```python
from build123d import *

# Parameters (mm, degrees)
SKETCH1_W          = 520
SKETCH1_H          = 192.12
BASE_FLANGE1_DEPTH = 3.26
SKETCH2_R          = 4.5
CUT_EXTRUDE1_DEPTH = 10
SKETCH3_R          = 2.5
CUT_EXTRUDE2_DEPTH = 10
SKETCH4_R          = 2.5
CUT_EXTRUDE3_DEPTH = 10
FILLET2_R          = 5
CHAMFER1_SIZE      = 2.5


# Sheet-metal steps are written as plain solids
with BuildPart() as part:
    # Sketch1 → Base-Flange1 (new body)
    with BuildSketch(Plane(origin=(0, 0, 0), x_dir=(1, 0, 0), z_dir=(0, 1, 0))):
        with Locations((0, -0.985)):
            Rectangle(SKETCH1_W, SKETCH1_H)
    extrude(amount=-BASE_FLANGE1_DEPTH)

    # Sketch2 → Cut-Extrude1 (cut)
    with BuildSketch(Plane(origin=(0, 0, 0), x_dir=(1, 0, 0), z_dir=(0, 1, 0))):
        with Locations(Location((130, 80.075, 0), (0, 0, 270))):
            Circle(SKETCH2_R)
        with Locations(Location((130, -82.545, 0), (0, 0, 270))):
            Circle(SKETCH2_R)
        with Locations(Location((-130, 80.075, 0), (0, 0, 270))):
            Circle(SKETCH2_R)
        with Locations(Location((-130, -82.545, 0), (0, 0, 270))):
            Circle(SKETCH2_R)
    extrude(amount=-CUT_EXTRUDE1_DEPTH, mode=Mode.SUBTRACT)

    # Sketch3 → Cut-Extrude2 (cut)
    with BuildSketch(Plane(origin=(0, 0, 0), x_dir=(1, 0, 0), z_dir=(0, 1, 0))):
        with Locations(Location((-52.5, 52.5, 0), (0, 0, 270))):
            Circle(SKETCH3_R)
        with Locations(Location((52.5, 52.5, 0), (0, 0, 270))):
            Circle(SKETCH3_R)
        with Locations(Location((52.5, -52.5, 0), (0, 0, 270))):
            Circle(SKETCH3_R)
        with Locations(Location((-52.5, -52.5, 0), (0, 0, 270))):
            Circle(SKETCH3_R)
        with BuildLine():
            Line((-3, -59.924953066), (-3, -19.773719933))
            ThreePointArc((-3, -19.773719933), (-7.653668647, -18.47759065), (-11.860811111, -16.103451798))
            Line((-11.860811111, -16.103451798), (-40.252020332, -44.494661019))
            ThreePointArc((-40.252020332, -44.494661019), (-22.961005942, -55.432771951), (-3, -59.924953066))
        make_face()
        with BuildLine():
            Line((-3, 59.924953066), (-3, 19.773719933))
            ThreePointArc((-3, 19.773719933), (-7.653668647, 18.47759065), (-11.860811111, 16.103451798))
            Line((-11.860811111, 16.103451798), (-40.252020332, 44.494661019))
            ThreePointArc((-40.252020332, 44.494661019), (-22.961005942, 55.432771951), (-3, 59.924953066))
        make_face()
        with BuildLine():
            Line((-19.773719933, 3), (-59.924953066, 3))
            ThreePointArc((-59.924953066, 3), (-55.432771951, 22.961005942), (-44.494661019, 40.252020332))
            Line((-44.494661019, 40.252020332), (-16.103451798, 11.860811111))
            ThreePointArc((-16.103451798, 11.860811111), (-18.47759065, 7.653668647), (-19.773719933, 3))
        make_face()
        with BuildLine():
            Line((-19.773719933, -3), (-59.924953066, -3))
            ThreePointArc((-59.924953066, -3), (-55.432771951, -22.961005942), (-44.494661019, -40.252020332))
            Line((-44.494661019, -40.252020332), (-16.103451798, -11.860811111))
            ThreePointArc((-16.103451798, -11.860811111), (-18.47759065, -7.653668647), (-19.773719933, -3))
        make_face()
        with BuildLine():
            Line((3, -59.924953066), (3, -19.773719933))
            ThreePointArc((3, -19.773719933), (7.653668647, -18.47759065), (11.860811111, -16.103451798))
            Line((11.860811111, -16.103451798), (40.252020332, -44.494661019))
            ThreePointArc((40.252020332, -44.494661019), (22.961005942, -55.432771951), (3, -59.924953066))
        make_face()
        with BuildLine():
            Line((44.494661019, -40.252020332), (16.103451798, -11.860811111))
            ThreePointArc((16.103451798, -11.860811111), (18.47759065, -7.653668647), (19.773719933, -3))
            Line((19.773719933, -3), (59.924953066, -3))
            ThreePointArc((59.924953066, -3), (55.432771951, -22.961005942), (44.494661019, -40.252020332))
        make_face()
        with BuildLine():
            Line((19.773719933, 3), (59.924953066, 3))
            ThreePointArc((59.924953066, 3), (55.432771951, 22.961005942), (44.494661019, 40.252020332))
            Line((44.494661019, 40.252020332), (16.103451798, 11.860811111))
            ThreePointArc((16.103451798, 11.860811111), (18.47759065, 7.653668647), (19.773719933, 3))
        make_face()
        with BuildLine():
            Line((40.252020332, 44.494661019), (11.860811111, 16.103451798))
            ThreePointArc((11.860811111, 16.103451798), (7.653668647, 18.47759065), (3, 19.773719933))
            Line((3, 19.773719933), (3, 59.924953066))
            ThreePointArc((3, 59.924953066), (22.961005942, 55.432771951), (40.252020332, 44.494661019))
        make_face()
    extrude(amount=-CUT_EXTRUDE2_DEPTH, mode=Mode.SUBTRACT)

    # Sketch4 → Cut-Extrude3 (cut)
    with BuildSketch(Plane(origin=(0, 0, 0), x_dir=(1, 0, 0), z_dir=(0, 1, 0))):
        with Locations(Location((-92.5, 52.5, 0), (0, 0, 270))):
            Circle(SKETCH4_R)
        with Locations(Location((-197.5, 52.5, 0), (0, 0, 270))):
            Circle(SKETCH4_R)
        with Locations(Location((-197.5, -52.5, 0), (0, 0, 270))):
            Circle(SKETCH4_R)
        with Locations(Location((-92.5, -52.5, 0), (0, 0, 270))):
            Circle(SKETCH4_R)
        with Locations(Location((92.5, -52.5, 0), (0, 0, 270))):
            Circle(SKETCH4_R)
        with Locations(Location((197.5, -52.5, 0), (0, 0, 270))):
            Circle(SKETCH4_R)
        with Locations(Location((197.5, 52.5, 0), (0, 0, 270))):
            Circle(SKETCH4_R)
        with Locations(Location((92.5, 52.5, 0), (0, 0, 270))):
            Circle(SKETCH4_R)
        Polygon((-100, 60), (-190, 60), (-190, 45), (-205, 45), (-205, -45), (-190, -45), (-190, -60), (-100, -60), (-100, -45), (-85, -45), (-85, 45), (-100, 45), align=None)
        Polygon((100, 45), (100, 60), (190, 60), (190, 45), (205, 45), (205, -45), (190, -45), (190, -60), (100, -60), (100, -45), (85, -45), (85, 45), align=None)
    extrude(amount=-CUT_EXTRUDE3_DEPTH, mode=Mode.SUBTRACT)

    # Fillet2
    fillet2_edges = [part.edges().sort_by_distance(p)[0] for p in [
        (-100, -1.63, -60),
        (-100, -1.63, -45),
        (-85, -1.63, -45),
        (-85, -1.63, 45),
        (-100, -1.63, 45),
        (-100, -1.63, 60),
        (-190, -1.63, 60),
        (-190, -1.63, 45),
        (-205, -1.63, 45),
        (-205, -1.63, -45),
        (-190, -1.63, -45),
        (-190, -1.63, -60),
        (85, -1.63, -45),
        (100, -1.63, -45),
        (100, -1.63, -60),
        (190, -1.63, -60),
        (190, -1.63, -45),
        (205, -1.63, -45),
        (205, -1.63, 45),
        (190, -1.63, 45),
        (190, -1.63, 60),
        (100, -1.63, 60),
        (100, -1.63, 45),
        (85, -1.63, 45),
    ]]
    fillet(fillet2_edges, radius=FILLET2_R)

    # Chamfer1
    chamfer1_edges = [part.edges().sort_by_distance(p)[0] for p in [
        (130, 0, -84.575),
        (130, 0, 78.045),
        (-130, 0, -84.575),
        (-130, 0, 78.045),
    ]]
    chamfer(chamfer1_edges, length=CHAMFER1_SIZE)


solid = part.part
```
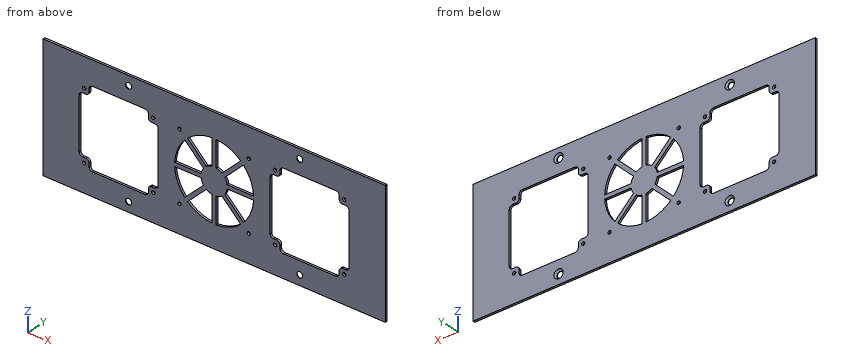
Here's how the part is built. I have some questions about the finished solid (model axes, mm). Coordinates: 2 decimals unless noted, no trailing zeros. Order: outer loops, then holes, each group sorted by start corner. A loop starts at its lowest first (then second) coordinate and runs counter-clockwise, first axis right, second up. Notation, with made-up numbers: (73, 25) -> (96, 25) arc R14 cw to (96, 34) -> close; hole circle Ø1 at (18.25, 21). An arc over 180 degrees is marked (long way). Return JSON: item names as keys, results as strings.
1) I'm going to push a flat-ended pin straight in: P1, Ø7, axis at x = 130, z = 82.545, coming from the -Y side. Where does the tip first touch, or does it pass through?
Conclusion:
{"P1": "passes through"}
2) If we section it at B-B on z = 26: List the corners of the cut face in (x, y) for me.
Conclusion:
{"outline": "(-260, -3.26) -> (-205, -3.26) -> (-205, 0) -> (-260, 0) -> close; (-85, -3.26) -> (-54.07, -3.26) -> (-54.07, 0) -> (-85, 0) -> close; (-30.24, -3.26) -> (-21.76, -3.26) -> (-21.76, 0) -> (-30.24, 0) -> close; (-3, -3.26) -> (3, -3.26) -> (3, 0) -> (-3, 0) -> close; (21.76, -3.26) -> (30.24, -3.26) -> (30.24, 0) -> (21.76, 0) -> close; (54.07, -3.26) -> (85, -3.26) -> (85, 0) -> (54.07, 0) -> close; (205, -3.26) -> (260, -3.26) -> (260, 0) -> (205, 0) -> close"}
3) If we section it at C-C on x = -130: List the corners of the cut face in (y, z) for me (3 decimals), plus the area to 3 significant figures.
Conclusion:
{"outline": "(-3.26, -95.075) -> (0, -95.075) -> (0, -87.075) -> (-2.5, -84.575) -> (-3.26, -84.575) -> close; (-3.26, -75.575) -> (-2.5, -75.575) -> (0, -73.075) -> (0, -60) -> (-3.26, -60) -> close; (-3.26, 60) -> (0, 60) -> (0, 75.545) -> (-2.5, 78.045) -> (-3.26, 78.045) -> close; (-3.26, 87.045) -> (-2.5, 87.045) -> (0, 89.545) -> (0, 97.045) -> (-3.26, 97.045) -> close", "area": "164 mm²"}
4) If we section it at A-A on x = 158.5: List the corners of the cut face in (y, z) for me (3 decimals).
Conclusion:
{"outline": "(-3.26, -95.075) -> (0, -95.075) -> (0, -60) -> (-3.26, -60) -> close; (-3.26, 60) -> (0, 60) -> (0, 97.045) -> (-3.26, 97.045) -> close"}
5) If I drill on probe 1 along Z at (x, y) = (197.5, -1.9) (3 decimals); probe 2 along X at (y, z) = (-2.4, -1.5); probe 3 along X at (y, z) = (-1.4, 84), over which ranges is the centre line in solid material (lowest first)?
Conclusion:
{"probe 1": "z = -95.075 to -55, -50 to -45, 45 to 50, 55 to 97.045", "probe 2": "x = -260 to -205, -85 to 85, 205 to 260", "probe 3": "x = -260 to -135.41, -124.59 to 124.59, 135.41 to 260"}
6) If we section it at D-D on x = 29.5: List the corners of the cut face in (y, z) for me (3 decimals).
Conclusion:
{"outline": "(-3.26, -95.075) -> (0, -95.075) -> (0, -52.247) -> (-3.26, -52.247) -> close; (-3.26, -33.743) -> (0, -33.743) -> (0, -25.257) -> (-3.26, -25.257) -> close; (-3.26, -3) -> (0, -3) -> (0, 3) -> (-3.26, 3) -> close; (-3.26, 25.257) -> (0, 25.257) -> (0, 33.743) -> (-3.26, 33.743) -> close; (-3.26, 52.247) -> (0, 52.247) -> (0, 97.045) -> (-3.26, 97.045) -> close"}
